```python
from build123d import *

# Parameters (mm, degrees)
BOSS_EXTRUDE1_DEPTH = 20
SKETCH3_R           = 3
BOSS_EXTRUDE3_DEPTH = 3
FILLET2_R           = 2


with BuildPart() as part:
    # Sketch1 → Boss-Extrude1 (new body)
    with BuildSketch(Plane.XY):
        with BuildLine():
            Line((0, 0), (-95, 0))
            ThreePointArc((-95, 0), (-98.535533906, 1.464466094), (-100, 5))
            Line((-100, 5), (-100, 25))
            ThreePointArc((-100, 25), (-98.535533906, 28.535533906), (-95, 30))
            Line((-95, 30), (0, 30))
            Line((0, 30), (0, 0))
        make_face()
    extrude(amount=BOSS_EXTRUDE1_DEPTH)

    # Sketch3 → Boss-Extrude3 (add)
    with BuildSketch(Plane(origin=(0, 0, 0), x_dir=(0, 0, -1), z_dir=(1, 0, 0))):
        with Locations(Location((-9, 22, 0), (0, 0, 180))):
            Circle(SKETCH3_R)
        with Locations(Location((-9, 8, 0), (0, 0, 180))):
            Circle(SKETCH3_R)
    extrude(amount=BOSS_EXTRUDE3_DEPTH)

    # Fillet2
    fillet2_edges = [part.edges().sort_by_distance(p)[0] for p in [
        (-98.535533906, 28.535533906, 20),
        (-100, 15, 20),
        (-98.535533906, 1.464466094, 20),
        (-47.5, 0, 20),
        (-47.5, 30, 20),
    ]]
    fillet(fillet2_edges, radius=FILLET2_R)


solid = part.part
```
Design review of the part built by this model. Coordinates are the model's own, in mm. Give positions to 0.01 mm unless a question says otherwise; leave off trailing zeros. Order: outer loops, then holes, each group sorted by start corner. A loop starts at its lowest first (then second) coordinate and runs counter-clockwise, first axis right, second up. Notation, with made-up numbers: (-17.75, -22.5) -> (-13.75, -22.5) arc R17 ccw to (-13.75, -8.5) -> close; hole circle Ø9 at (-4, -20). An arc over 180 degrees is marked (long way). Write item = value, one per line. Start each with the question number.
(1) We need section A-A on z = 9. Write out the cut boundary in (x, y).
(2) We need section B-B on y = 22. Write out the cut boundary in (x, z), plus the area to 3 significant figures.
(3) To check wall thickness, follow line 1 along X through (y, z) = (14.5, 6.75); line 2 along X through (y, z) = (2.75, 12.75); line 3 along Y through (x, z) = (-63, 19.25). State the ranges of each line that lie inside material, in increasing order.
(4) We need section D-D on y = 6.75. Write out the cut boundary in (x, z), plus the area to 3 significant figures.
(5) For pin 1 (1 mm diameter, centred on y = 21, z = 3.5, fed in from +X); pin 2 (10 mm diameter, centred on y = 8, z = 12.5, fed in from +X), all flat-tipped, find the tip position at first contact; note any pin that passes through.
(6) We need section C-C on z = 15.5. Write out the cut boundary in (x, y).
(7) Mouldability with a two-part tool opening along Y and no side actions: class faces 1 (the face through (1.479, 24.662, 10.384)), 2 (the face through (-100, 15, 9)), 3 (the face through (-48.16, 0.6, 19.43)), 4 (the face through (1.48, 7.1, 11.86)) as +Y half, -Y half, draft (parallel to the pull), parting line (faces both ways), or undercut.
Numbers:
q1.outline = (-100, 5) arc R5 ccw to (-95, 0) -> (0, 0) -> (0, 5) -> (3, 5) -> (3, 11) -> (0, 11) -> (0, 19) -> (3, 19) -> (3, 25) -> (0, 25) -> (0, 30) -> (-95, 30) arc R5 ccw to (-100, 25) -> close
q2.outline = (-100, 0) -> (0, 0) -> (0, 6) -> (3, 6) -> (3, 12) -> (0, 12) -> (0, 20) -> (-98, 20) arc R2 ccw to (-100, 18) -> close
q2.area = 2,020 mm^2
q3.line_1 = -100 to 0
q3.line_2 = -99.47 to 0
q3.line_3 = 0.44 to 29.56
q4.outline = (-100, 0) -> (0, 0) -> (0, 6.27) -> (3, 6.27) -> (3, 11.73) -> (0, 11.73) -> (0, 20) -> (-98, 20) arc R2 ccw to (-100, 18) -> close
q4.area = 2,020 mm^2
q5.pin_1 = 0
q5.pin_2 = 3
q6.outline = (-100, 5) arc R5 ccw to (-95, 0) -> (0, 0) -> (0, 30) -> (-95, 30) arc R5 ccw to (-100, 25) -> close
q7.face_1 = undercut
q7.face_2 = draft
q7.face_3 = -Y half
q7.face_4 = undercut
